from build123d import *

# Parameters (mm, degrees)
SKETCH_W      = 60
SKETCH_H      = 3
PAD_DEPTH     = 35
SKETCH001_R   = 1.5
SKETCH001_R_2 = 2
SKETCH001_R_3 = 2.5
SKETCH001_W   = 5
SKETCH001_H   = 5
POCKET_DEPTH  = 3


with BuildPart() as part:
    # Sketch → Pad (new body)
    with BuildSketch(Plane.XY):
        with Locations((30, 1.5)):
            Rectangle(SKETCH_W, SKETCH_H)
    extrude(amount=PAD_DEPTH)

    # Sketch001 → Pocket (cut)
    with BuildSketch(Plane.XZ):
        with Locations((20, 10)):
            Circle(SKETCH001_R)
        with Locations((26, 10)):
            Circle(SKETCH001_R_2)
        with Locations((20, 16)):
            Circle(SKETCH001_R_2)
        with Locations((14, 10)):
            Circle(SKETCH001_R_2)
        with Locations((20, 4)):
            Circle(SKETCH001_R_2)
        with Locations((5, 30)):
            Circle(SKETCH001_R_3)
        with Locations((55, 30)):
            Circle(SKETCH001_R_3)
        with Locations((22.5, 30)):
            Rectangle(SKETCH001_W, SKETCH001_H)
        with Locations((37.5, 30)):
            Rectangle(SKETCH001_W, SKETCH001_H)
    extrude(amount=-POCKET_DEPTH, mode=Mode.SUBTRACT)


solid = part.part
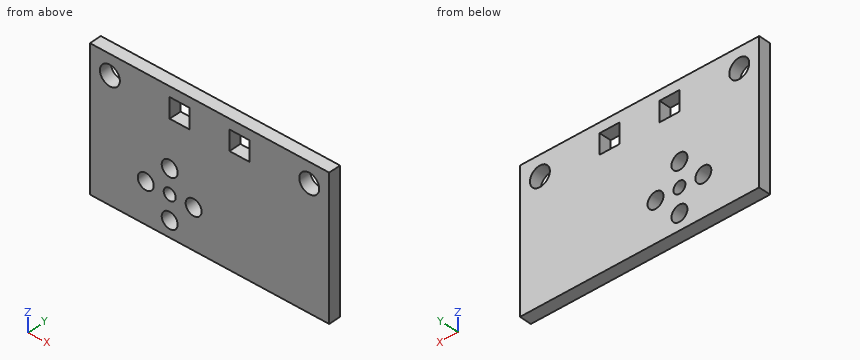
Check sheet for the modelled part. Datum: model origin and axes. Units: mm. Give positions to 0.01 mm unless a question says otherwise; leave off trailing zeros. Loops run counter-clockwise (first coordinate to the right, second up) from the corner with the lowest first, then second, coordinate; pieces in that order, holes last. Notation, with made-up numbers: M -33.75,26.5 L -22.75,26.5 A15 cw -22.75,40.5 Z; hole C 50,82 d3. An arc over 180 degrees is marked long. Use a Markdown table: item, result. Add a question column.
Q1. Sectioned sample at D-D, the plane z = 10. Record the cut outline in (x, y).
Q2. Go/stop test with flat-tipped pins: pin 1 (0.9 mm diameter, centred on y = 1.5, z = 30.5, fed in from -X); pin 2 (3.5 mm diameter, centred on x = 26, z = 10, fed in from -Y) (3 decimals). Record where each tip stops, or that it passes through.
Q3. Scan lines: line 1 along Z through (x, y) = (14, 2.45); line 2 along X through (y, z) = (1.5, 32); line 3 along Z through (x, y) = (55, 1.65). Record each from-to range of solid material in increasing order. Write a range as [from, to].
Q4. Sectioned sample at B-B, the plane x = 26. Record the cut outline in (y, z).
Q5. Sectioned sample at A-A, the plane z = 16. Record the cut outline in (x, y), then the cut area to 3 significant figures.
Q6. Sectioned sample at C-C, the plane y = 0.45. Give the number of separate pieces and of enclosed holes in the cut face, then the cut area to 3 significant figures.
Verdict:
| question | item | result |
|---|---|---|
| 1 | outline | M 0,0 L 12,0 L 12,3 L 0,3 Z; M 16,0 L 18.5,0 L 18.5,3 L 16,3 Z; M 21.5,0 L 24,0 L 24,3 L 21.5,3 Z; M 28,0 L 60,0 L 60,3 L 28,3 Z |
| 2 | pin 1 | x = 0 |
| 2 | pin 2 | through |
| 3 | line 1 | [0, 8], [12, 35] |
| 3 | line 2 | [0, 3.5], [6.5, 20], [25, 35], [40, 53.5], [56.5, 60] |
| 3 | line 3 | [0, 27.5], [32.5, 35] |
| 4 | outline | M 0,0 L 3,0 L 3,8 L 0,8 Z; M 0,12 L 3,12 L 3,35 L 0,35 Z |
| 5 | outline | M 0,0 L 18,0 L 18,3 L 0,3 Z; M 22,0 L 60,0 L 60,3 L 22,3 Z |
| 5 | area | 168 mm^2 |
| 6 | separate pieces | 1 |
| 6 | enclosed holes | 9 |
| 6 | area | 1,950 mm^2 |
